Check sheet for the drawn part. Datum: minimum x, y, z corner. Units: mm. A direction names the side the tool comes from. Round coordinates to 2 decimals unless told otherwise and drop trailing zeros. Write each loop counter-clockwise with the first axis right and the second up, starting at its lowest first coordinate (ties: lowest second). Pieces come first, ordered by that corner, then holes. Notation, with made-up numbers: (-38.75, -36.75) - (20.25, -36.75) arc R24 cw to (20.25, -23.75) - close; hole circle Ø7 at (84, 75). An arc over 180 degrees is marked (long way). Answer as a JSON object with one key per item and string values.
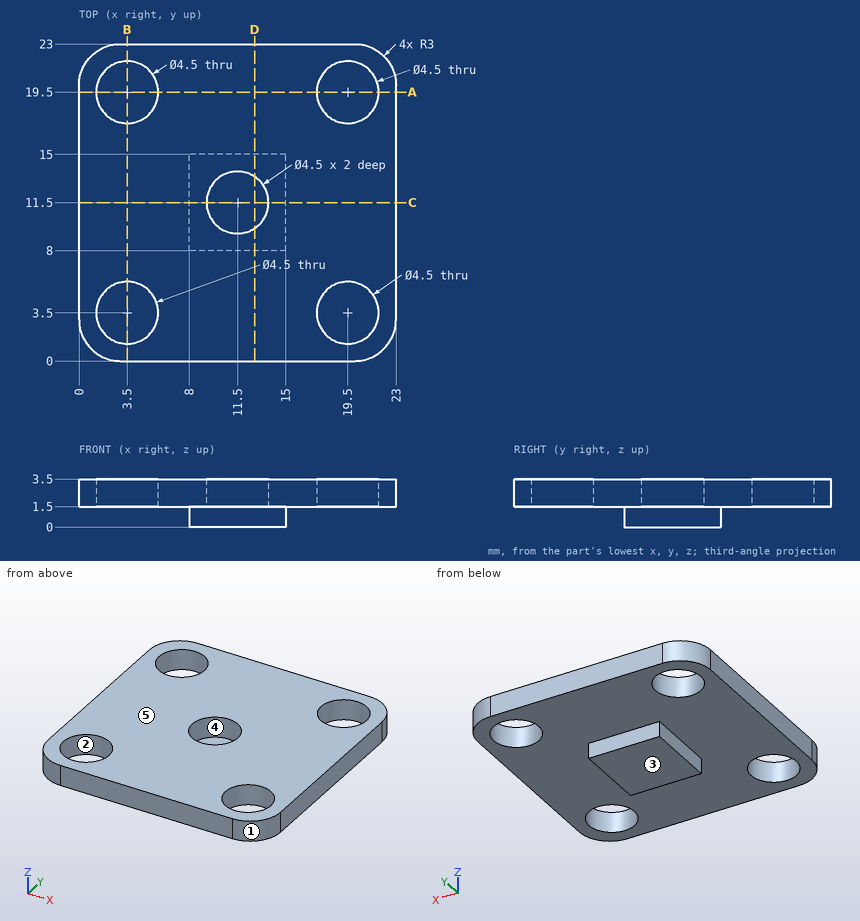
1. Cross-section at D-D (x = 12.75). Record the boundary of the cut face in (y, z), plus the area to 3 significant figures.
Completed:
{"outline": "(0, 1.5) - (8, 1.5) - (8, 0) - (15, 0) - (15, 1.5) - (23, 1.5) - (23, 3.5) - (13.37, 3.5) - (13.37, 1.5) - (9.63, 1.5) - (9.63, 3.5) - (0, 3.5) - close", "area": "49.0 mm^2"}
2. Go/stop test with flat-tipped pins: pin 1 (0.8 mm diameter, centred on x = 13, z = 1, fed in from +Y); pin 2 (6 mm diameter, centred on x = 11.5, y = 11.5, fed in from -Z); pin 3 (1 mm diameter, centred on y = 11, z = 0.5, fed in from -X); pin 4 (1.6 mm diameter, centred on x = 11, z = 0.5, fed in from -Y). Record where each tip stops, or that it passes through.
Completed:
{"pin 1": "stops at y = 15", "pin 2": "stops at z = 0", "pin 3": "stops at x = 8", "pin 4": "stops at y = 8"}
3. Material ranges on probe 1 along Y at (x, z) = (19.5, 2.3); probe 2 along Y at (x, z) = (1.5, 3.05); probe 3 along X at (y, z) = (20.75, 2.9), recorded low to high. Write a range as from..to.
Completed:
{"probe 1": "y = 0..1.25, 5.75..17.25, 21.75..23", "probe 2": "y = 0.4..2.47, 4.53..18.47, 20.53..22.6", "probe 3": "x = 0.1..1.63, 5.37..17.63, 21.37..22.9"}
4. Cross-section at C-C (y = 11.5). Record the boundary of the cut face in (x, z), plus the area to 3 significant figures.
Completed:
{"outline": "(0, 1.5) - (8, 1.5) - (8, 0) - (15, 0) - (15, 1.5) - (23, 1.5) - (23, 3.5) - (13.75, 3.5) - (13.75, 1.5) - (9.25, 1.5) - (9.25, 3.5) - (0, 3.5) - close", "area": "47.5 mm^2"}
5. Cross-section at A-A (y = 19.5). Record the boundary of the cut face in (x, z).
Completed:
{"outline": "(0, 1.5) - (1.25, 1.5) - (1.25, 3.5) - (0, 3.5) - close; (5.75, 1.5) - (17.25, 1.5) - (17.25, 3.5) - (5.75, 3.5) - close; (21.75, 1.5) - (23, 1.5) - (23, 3.5) - (21.75, 3.5) - close"}
6. Access from +Z, -Z, +X, -X, +Y, -Y to the whole of each face (thin tool, end or side, straight path). Record for the marked faces 4 and 5.
Completed:
{"face 4": "+Z", "face 5": "+Z, +X, -X, +Y, -Y"}
7. Mould release check, pull along X, two halves, no side actions. Record for the marked faces 1, 2 and 3: released by +X, released by -X, zero draft, split by the parting line, or undercut.
Completed:
{"face 1": "released by +X", "face 2": "undercut", "face 3": "zero draft"}
